from build123d import *

# Parameters (mm, degrees)
SKETCH_1_W          = 25
SKETCH_1_H          = 10
SKETCH_2_R          = 4
CUT_EXTRUDE_1_DEPTH = 8.5


with BuildPart() as part:
    # 草图1 → 旋转1 (revolve)
    with BuildSketch(Plane.XY, mode=Mode.PRIVATE) as revolve_1_sk:
        with Locations((0, 5)):
            Rectangle(SKETCH_1_W, SKETCH_1_H)
    revolve(revolve_1_sk.sketch.rotate(Axis((-12.5, 0, 0), (1, 0, 0)), 90), axis=Axis((-12.5, 0, 0), (1, 0, 0)))

    # 草图2 → 切除-拉伸1 (cut)
    with BuildSketch(Plane(origin=(12.5, 0, 0), x_dir=(0, 0, -1), z_dir=(1, 0, 0))):
        Circle(SKETCH_2_R)
    cut_extrude_1 = extrude(amount=-CUT_EXTRUDE_1_DEPTH, mode=Mode.SUBTRACT)

    # 镜向1: 切除-拉伸1 across plane
    add(cut_extrude_1.mirror(Plane(origin=(0, 0, 0), x_dir=(0, 0, 1), z_dir=(1, 0, 0))), mode=Mode.SUBTRACT)


solid = part.part
Input: part model. Units: mm. Frame: model coordinates. A direction names the side the tool comes from. Coordinates: 2 decimals unless noted, no trailing zeros. Loops run counter-clockwise (first coordinate to the right, second up) from the corner with the lowest first, then second, coordinate; pieces in that order, holes last. Notation, with made-up numbers: (9, -30) - (24, -30) arc R5 cw to (24, -24) - close; hole circle Ø4 at (29, -24). An arc over 180 degrees is marked (long way). Answer in a Markdown table with one row per item. Add a question column.
Item 1: Mould query, pull axis Z, two halves, no side actions, for faces 1 (the flat face through (4, 0, 0)), 2 (the flat face through (-12.5, -0.1, -4.3)), 3 (the cylindrical face through (0, 0, -10)). Classes: released by +Z, released by -Z, zero draft, split by the parting line, or undercut.
Item 2: Section query C-C on x = 7. Return the cut outline in (y, z).
Item 3: Contact query for flat-ended pins moving along their axis: P1, Ø2.5, axis at y = -1, z = 1, coming from the +X side; P2, Ø4, axis at x = 2, z = -2.5, coming from the -Y side; P3, Ø3, axis at x = -2.5, z = -4, coming from the -Y side. Output: stop coordinate, or through.
Item 4: Access query for faces 4 (the cylindrical face through (8.31, -3.905, 0.867)), 5 (the flat face through (12.5, -0.1, -4.3)), 6 (the flat face through (-4, 0, 0)). Directions: +Z, -Z, +X, -X, +Y, -Y. A direction counts if a zero-diameter tool reaches every point of the face in a straight line with its end or side. Return the directions, or none.
Item 5: Line query: line 1 along Y through (x, z) = (-9.25, 0); line 2 along Y through (x, z) = (5, -2); line 3 along Y through (x, z) = (-1.25, -7.75). Output: solid intervals per line, ascending. Write a range as [from, to].
Item 6: Section query D-D on x = -3.5. Return the cut outline in (y, z), then the cut area to 3 significant figures.
Item 7: Section query A-A on z = 0. Return the cut outline in (x, y), then the cut area to 3 significant figures.
Recorded:
| question | item | result |
|---|---|---|
| 1 | face 1 | undercut |
| 1 | face 2 | zero draft |
| 1 | face 3 | split by the parting line |
| 2 | outline | circle Ø20 at (0, 0); hole circle Ø8 at (0, 0) |
| 3 | P1 | x = 4 |
| 3 | P2 | y = -9.99 |
| 3 | P3 | y = -9.68 |
| 4 | face 4 | +X |
| 4 | face 5 | +Z, -Z, +X, +Y, -Y |
| 4 | face 6 | -X |
| 5 | line 1 | [-10, -4], [4, 10] |
| 5 | line 2 | [-9.8, -3.46], [3.46, 9.8] |
| 5 | line 3 | [-6.32, 6.32] |
| 6 | outline | circle Ø20 at (0, 0) |
| 6 | area | 314 mm^2 |
| 7 | outline | (-12.5, -10) - (12.5, -10) - (12.5, -4) - (4, -4) - (4, 4) - (12.5, 4) - (12.5, 10) - (-12.5, 10) - (-12.5, 4) - (-4, 4) - (-4, -4) - (-12.5, -4) - close |
| 7 | area | 364 mm^2 |
